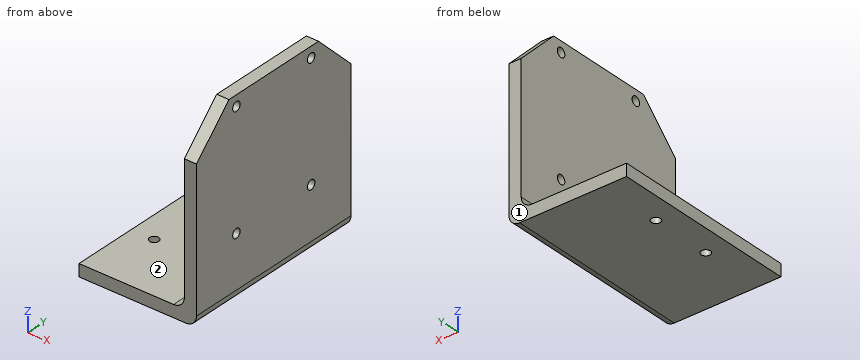
```python
from build123d import *

# Parameters (mm, degrees)
EXTRUDE_1_DEPTH     = 31
SKETCH_2_R          = 1.5
CUT_EXTRUDE_2_DEPTH = 10
FILLET_1_R          = 3.5
FILLET_2_R          = 3.5
SKETCH_7_R          = 1.5
CUT_EXTRUDE_4_DEPTH = 10


with BuildPart() as part:
    # 草图1 → 凸台-拉伸1 (new, symmetric)
    with BuildSketch(Plane(origin=(0, 0, 0), x_dir=(1, 0, 0), z_dir=(0, 1, 0))):
        Polygon((-27.626027397, 43.157534247), (10.873972603, 43.157534247), (10.873972603, -18.842465753), (6.873972603, -18.842465753), (6.873972603, 39.157534247), (-27.626027397, 39.157534247), align=None)
    extrude(amount=EXTRUDE_1_DEPTH, both=True)

    # 草图2 → 切除-拉伸2 (cut)
    with BuildSketch(Plane(origin=(10.873972603, 0, 0), x_dir=(0, 0, -1), z_dir=(1, 0, 0))):
        Polygon((-5.842465753, 31), (-18.842465753, 31), (-18.842465753, 18), align=None)
        with Locations((22.657534247, -15)):
            Circle(SKETCH_2_R)
        Polygon((-5.842465753, -31), (-18.842465753, -18), (-18.842465753, -31), align=None)
        with Locations((22.657534247, 15)):
            Circle(SKETCH_2_R)
        with Locations((-15.342465753, 15)):
            Circle(SKETCH_2_R)
        with Locations((-15.342465753, -15)):
            Circle(SKETCH_2_R)
    extrude(amount=-CUT_EXTRUDE_2_DEPTH, mode=Mode.SUBTRACT)

    # 圆角1
    fillet_1_edges = [part.edges().sort_by_distance(p)[0] for p in [
        (10.873972603, 0, -43.157534247),
    ]]
    fillet(fillet_1_edges, radius=FILLET_1_R)

    # 圆角2
    fillet_2_edges = [part.edges().sort_by_distance(p)[0] for p in [
        (6.873972603, 0, -39.157534247),
    ]]
    fillet(fillet_2_edges, radius=FILLET_2_R)

    # 草图7 → 切除-拉伸4 (cut)
    with BuildSketch(Plane(origin=(0, 0, -43.157534247), x_dir=(-1, 0, 0), z_dir=(0, 0, -1))):
        with Locations((20.126027397, 10)):
            Circle(SKETCH_7_R)
        with Locations((20.126027397, -10)):
            Circle(SKETCH_7_R)
    extrude(amount=-CUT_EXTRUDE_4_DEPTH, mode=Mode.SUBTRACT)


solid = part.part
```
Verification items for the finished model (mm, model axes). Face numbers are marked on the shaded views. A direction names the side the tool comes from. Round coordinates to 2 decimals unless told otherwise and drop trailing zeros. Write each loop counter-clockwise with the first axis right and the second up, starting at its lowest first coordinate (ties: lowest second). Pieces come first, ordered by that corner, then holes.
1. Section check D-D on z = -20. Enter the section's corners in (x, y), plus the area to 3 significant figures.
2. Section check C-C on y = 20. Enter the section's corners in (x, z).
3. Section check A-A on y = 10. Enter the section's corners in (x, z), plus the area to 3 significant figures.
4. Gauge pin test, flat ends, axial feed: P1, Ø4, axis at x = -1, y = -18.5, coming from the +Z side; P2, Ø2.5, axis at x = -20.13, y = -10, coming from the -Z side; P3, Ø5, axis at y = -15, z = 15.34, coming from the +X side; P4, Ø4, axis at y = 15, z = -22.66, coming from the -X side. Record the tip position at first contact, or that the pin passes through.
5. Section check B-B on y = -15. Enter the section's corners in (x, z).
6. Access from +Z, -Z, +X, -X, +Y, -Y to the whole of each face (thin tool, end or side, straight path). Record for the marked faces 1 and 2.
7. Scan lines: L1, parallel to Y at x = -20, z = -40; L2, parallel to Z at x = -18, y = -2; L3, parallel to X at y = 0.5, z = 11.5. Record each from-to range of solid material in increasing order.
Answer:
1. outline: (6.87, -31) - (10.87, -31) - (10.87, 31) - (6.87, 31) - close
1. area: 248 mm2
2. outline: (-27.63, -43.16) - (7.37, -43.16) arc R3.5 ccw to (10.87, -39.66) - (10.87, 16.84) - (6.87, 16.84) - (6.87, -35.66) arc R3.5 cw to (3.37, -39.16) - (-27.63, -39.16) - close
3. outline: (-27.63, -43.16) - (-21.63, -43.16) - (-21.63, -39.16) - (-27.63, -39.16) - close; (-18.63, -43.16) - (7.37, -43.16) arc R3.5 ccw to (10.87, -39.66) - (10.87, 18.84) - (6.87, 18.84) - (6.87, -35.66) arc R3.5 cw to (3.37, -39.16) - (-18.63, -39.16) - close
3. area: 374 mm2
4. P1: stops at z = -39.16
4. P2: passes through
4. P3: stops at x = 10.87
4. P4: stops at x = 6.87
5. outline: (-27.63, -43.16) - (7.37, -43.16) arc R3.5 ccw to (10.87, -39.66) - (10.87, -24.16) - (6.87, -24.16) - (6.87, -35.66) arc R3.5 cw to (3.37, -39.16) - (-27.63, -39.16) - close; (6.87, -21.16) - (10.87, -21.16) - (10.87, 13.84) - (6.87, 13.84) - close; (6.87, 16.84) - (10.87, 16.84) - (10.87, 18.84) - (6.87, 18.84) - close
6. face 1: +Z, -Z, +X, -X, +Y
6. face 2: +Z, -X, +Y, -Y
7. L1: y = -31 to -11.49, -8.51 to 8.51, 11.49 to 31
7. L2: z = -43.16 to -39.16
7. L3: x = 6.87 to 10.87
